Geometry check sheet. Reference: drawing and pictorial views, mm from the part's lowest x, y, z. Coordinates: 2 decimals unless noted, no trailing zeros. Write each loop counter-clockwise with the first axis right and the second up, starting at its lowest first coordinate (ties: lowest second). Pieces come first, ordered by that corner, then holes.
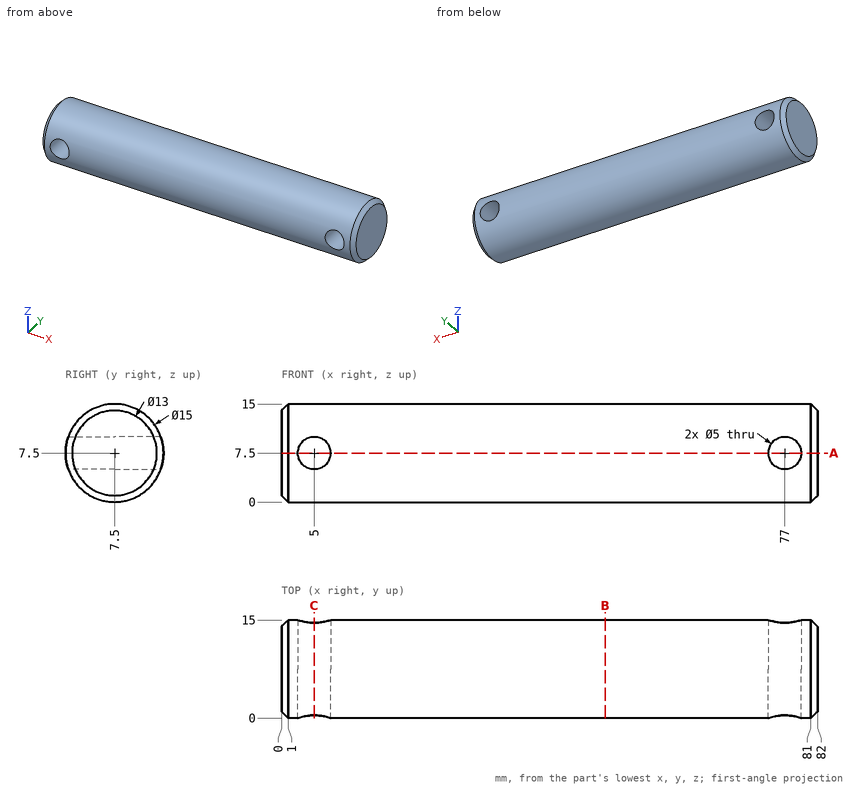
1. Gauge pin test, flat ends, axial feed: P1, Ø3, axis at x = 77, z = 7.5, coming from the +Y side; P2, Ø1.5, axis at x = 19.5, z = 10.5, coming from the -Y side; P3, Ø6, axis at x = 13.5, z = 4, coming from the +Y side; P4, Ø1, axis at x = 32, y = 13, coming from the +Z side. Record the tip position at first contact, or that the pin passes through.
2. Material ranges on L1, parallel to X at y = 3.75, z = 7.5; L2, parallel to X at y = 8.5, z = 6.5; L3, parallel to Z at x = 5, y = 9.75, recorded low to high.
3. Sectioned sample at A-A, the plane z = 7.5. Record the boundary of the cut face in (x, y), and give its area (3 significant figures).
4. Sectioned sample at C-C, the plane x = 5. Record the boundary of the cut face in (y, z).
5. Sectioned sample at B-B, the plane x = 49.5. Record the boundary of the cut face in (y, z), and give its area (3 significant figures).
Outcome:
1. P1: passes through
1. P2: stops at y = 0.35
1. P3: stops at y = 14.98
1. P4: stops at z = 13.09
2. L1: x = 0 to 2.5, 7.5 to 74.5, 79.5 to 82
2. L2: x = 0 to 2.71, 7.29 to 74.71, 79.29 to 82
2. L3: z = 0.35 to 5, 10 to 14.65
3. outline: (0, 1) - (1, 0) - (2.5, 0) - (2.5, 15) - (1, 15) - (0, 14) - close; (7.5, 0) - (74.5, 0) - (74.5, 15) - (7.5, 15) - close; (79.5, 0) - (81, 0) - (82, 1) - (82, 14) - (81, 15) - (79.5, 15) - close
3. area: 1,080 mm2
4. outline: (0.43, 5) arc R7.5 ccw to (14.57, 5) - close; (0.43, 10) - (14.57, 10) arc R7.5 ccw to start
5. outline: circle Ø15 at (7.5, 7.5)
5. area: 177 mm2
